Build history of the part. All positions in model axes, mm. Round coordinates to 2 decimals unless told otherwise and drop trailing zeros. Order: outer loops, then holes, each group sorted by start corner. A loop starts at its lowest first (then second) coordinate and runs counter-clockwise, first axis right, second up. Notation, with made-up numbers: M 16,-29.5 L 30,-29.5 A34 ccw 30,5.5 Z; hole C 69.5,-16 d8. An arc over 180 degrees is marked long. Use CSV: the item, a comma, the result in double quotes.
from build123d import *

# Parameters (mm, degrees)
SKETCH_1_W          = 20
SKETCH_1_H          = 40
SKETCH_1_W_2        = 50
SKETCH_1_H_2        = 20
EXTRUDE_1_DEPTH     = 3
SKETCH_2_R          = 2
CUT_EXTRUDE_1_DEPTH = 10
EXTRUDE_2_DEPTH     = 3


with BuildPart() as part:
    # 草图1 → 凸台-拉伸1 (new body)
    with BuildSketch(Plane.XY):
        with Locations((-20, -50)):
            Rectangle(SKETCH_1_W, SKETCH_1_H)
        with BuildLine():
            Line((-10, -30), (-10, -70))
            Line((-10, -70), (1, -70))
            Line((1, -70), (1, -67))
            ThreePointArc((1, -67), (-1.5, -64.5), (1, -62))
            Line((1, -62), (1, -33))
            ThreePointArc((1, -33), (-0.947653554, -32.067369017), (-1.442153468, -29.965316507))
            ThreePointArc((-1.442153468, -29.965316507), (-5.782490578, -29.437438793), (-10, -28.284271247))
            Line((-10, -28.284271247), (-10, -30))
        make_face()
        with BuildLine():
            Line((1, -67), (1, -70))
            Line((1, -70), (12, -70))
            Line((12, -70), (12, -27.49545417))
            ThreePointArc((12, -27.49545417), (7.787152469, -28.971714765), (3.401885012, -29.806495573))
            ThreePointArc((3.401885012, -29.806495573), (3.475349726, -30.149794724), (3.5, -30.5))
            ThreePointArc((3.5, -30.5), (2.767766953, -32.267766953), (1, -33))
            Line((1, -33), (1, -62))
            ThreePointArc((1, -62), (2.767766953, -62.732233047), (3.5, -64.5))
            ThreePointArc((3.5, -64.5), (2.767766953, -66.267766953), (1, -67))
        make_face()
        with BuildLine():
            Line((-10, -25), (-10, -28.284271247))
            ThreePointArc((-10, -28.284271247), (-5.782490578, -29.437438793), (-1.442153468, -29.965316507))
            ThreePointArc((-1.442153468, -29.965316507), (-0.567369017, -28.552346446), (1, -28))
            Line((1, -28), (1, -25))
            Line((1, -25), (-10, -25))
        make_face()
        with BuildLine():
            ThreePointArc((3.401885012, -29.806495573), (7.787152469, -28.971714765), (12, -27.49545417))
            Line((12, -27.49545417), (12, -25))
            Line((12, -25), (1, -25))
            Line((1, -25), (1, -28))
            ThreePointArc((1, -28), (2.502704052, -28.502030898), (3.401885012, -29.806495573))
        make_face()
        with BuildLine():
            Line((-30, -10), (-30, -30))
            Line((-30, -30), (-10, -30))
            Line((-10, -30), (-10, -28.284271247))
            ThreePointArc((-10, -28.284271247), (-21.213203436, -21.213203436), (-28.284271247, -10))
            Line((-28.284271247, -10), (-30, -10))
        make_face()
        with BuildLine():
            ThreePointArc((-28.284271247, -10), (-21.213203436, -21.213203436), (-10, -28.284271247))
            Line((-10, -28.284271247), (-10, -25))
            Line((-10, -25), (-10, -10))
            Line((-10, -10), (-28.284271247, -10))
        make_face()
        with Locations((-55, -20)):
            Rectangle(SKETCH_1_W_2, SKETCH_1_H_2)
    extrude(amount=EXTRUDE_1_DEPTH)

    # 草图2 → 切除-拉伸1 (cut)
    with BuildSketch(Plane(origin=(0, 0, 0), x_dir=(-1, 0, 0), z_dir=(0, 0, -1))):
        with Locations((20, -40)):
            Circle(SKETCH_2_R)
        with Locations((40, -20)):
            Circle(SKETCH_2_R)
        with Locations((20, -20)):
            Circle(SKETCH_2_R)
        with Locations((20, -60)):
            Circle(SKETCH_2_R)
        with Locations((60, -20)):
            Circle(SKETCH_2_R)
    extrude(amount=-CUT_EXTRUDE_1_DEPTH, mode=Mode.SUBTRACT)

    # 草图3 → 凸台-拉伸2 (add)
    with BuildSketch(Plane.XY.offset(3)):
        with BuildLine():
            Line((-10, -25), (12, -25))
            ThreePointArc((12, -25), (3.597916023, -13.689723166), (-10, -10))
            Line((-10, -10), (-10, -25))
        make_face()
    extrude(amount=-EXTRUDE_2_DEPTH)


solid = part.part
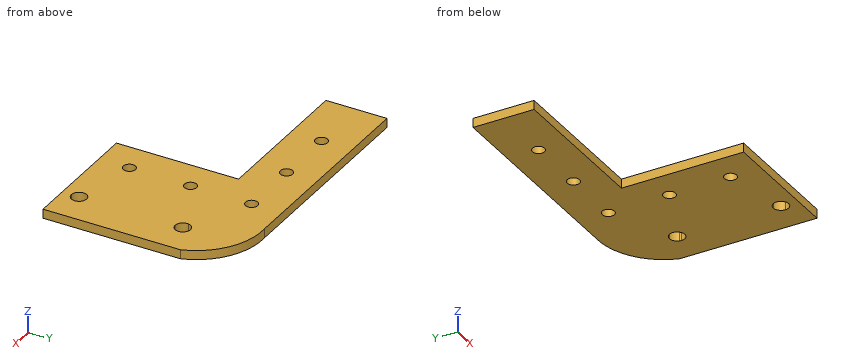
(1) Cut at A-A, the plane y = -40. Give the cut face in (x, z), and give its area (3 significant figures).
Answer block:
outline,"M -30,0 L -22,0 L -22,3 L -30,3 Z; M -18,0 L 12,0 L 12,3 L -18,3 Z"
area,"114 mm²"
(2) Cut at D-D, the plane x = -21. Give the cut face in (y, z), and give its area (3 significant figures).
Answer block:
outline,"M -70,0 L -61.73,0 L -61.73,3 L -70,3 Z; M -58.27,0 L -41.73,0 L -41.73,3 L -58.27,3 Z; M -38.27,0 L -21.73,0 L -21.73,3 L -38.27,3 Z; M -18.27,0 L -10,0 L -10,3 L -18.27,3 Z"
area,"149 mm²"
(3) Cut at B-B, the plane z = 0.45. Give the cut face in (x, y), and give its area (3 significant figures).
Answer block:
outline,"M -80,-30 L -30,-30 L -30,-70 L 12,-70 L 12,-25 A21.52 ccw -10,-10 L -80,-10 Z; hole C -60,-20 d4; hole C -40,-20 d4; hole C -20,-60 d4; hole C -20,-40 d4; hole C -20,-20 d4; hole C 1,-64.5 d5; hole C 1,-30.5 d5"
area,"3,340 mm²"
(4) Cut at C-C, the plane x = -60. Give the cut face in (y, z).
Answer block:
outline,"M -30,0 L -22,0 L -22,3 L -30,3 Z; M -18,0 L -10,0 L -10,3 L -18,3 Z"
(5) Wall check: line 1 (Y direction, x = -20, z = 2.4); line 2 (Y direction, x = -60, z = 1.9); line 3 (Y direction, x = -72, z = 0.65). Give the ranges that are in metal, low to high. Write a range as from..to.
Answer block:
line 1,"y = -70..-62, -58..-42, -38..-22, -18..-10"
line 2,"y = -30..-22, -18..-10"
line 3,"y = -30..-10"
(6) Drop flat-ended pins along their axis: pin 1 (1.5 mm diameter, centred on x = -47.5, z = 2, fed in from +Y); pin 2 (3.5 mm diameter, centred on x = -20, y = -40, fed in from -Z) (1 decimal); pin 3 (4.5 mm diameter, centred on x = -20, y = -60, fed in from +Z). Give the stop position or say it passes through.
Answer block:
pin 1,"stops at y = -10"
pin 2,"passes through"
pin 3,"stops at z = 3"
